Could you check a few things on this model? Use its own coordinates, in mm. A direction names the side the tool comes from. Coordinates: 2 decimals unless noted, no trailing zeros. Write each loop counter-clockwise with the first axis right and the second up, starting at its lowest first coordinate (ties: lowest second). Pieces come first, ordered by that corner, then holes.
```python
from build123d import *

# Parameters (mm, degrees)
F1_DEPTH = 1.2
F2_DEPTH = 2.2


with BuildPart() as f1:
    # F0 (on Top) → F1 (new body)
    with BuildSketch(Plane.XY):
        with BuildLine():
            ThreePointArc((-2.61423, 14.119491), (-10.150846, 10.145596), (-14.120842, 2.606925))
            Line((-14.120842, 2.606925), (-12.54888, 2.308583))
            ThreePointArc((-12.54888, 2.308583), (-12.746063, 0.003032), (-12.549977, -2.302612))
            Line((-12.549977, -2.302612), (-14.122546, -2.597676))
            ThreePointArc((-14.122546, -2.597676), (-10.138682, -10.128644), (-2.611663, -14.119966))
            Line((-2.611663, -14.119966), (-2.320738, -12.546638))
            ThreePointArc((-2.320738, -12.546638), (0.002028, -12.751949), (2.324728, -12.545899))
            Line((2.324728, -12.545899), (2.616123, -14.119141))
            ThreePointArc((2.616123, -14.119141), (10.123734, -10.218797), (14.094074, -2.747967))
            Line((14.094074, -2.747967), (12.522112, -2.449625))
            ThreePointArc((12.522112, -2.449625), (12.759115, -0.023547), (12.531068, 2.40339))
            Line((12.531068, 2.40339), (14.103637, 2.698454))
            ThreePointArc((14.103637, 2.698454), (10.129638, 10.19315), (2.610249, 14.120228))
            Line((2.610249, 14.120228), (2.319324, 12.546899))
            ThreePointArc((2.319324, 12.546899), (-0.001785, 12.754501), (-2.322835, 12.54625))
            Line((-2.322835, 12.54625), (-2.61423, 14.119491))
        make_face()
    extrude(amount=F1_DEPTH)

    # F0 (on Top) → F2 (join)
    with BuildSketch(Plane.XY):
        with BuildLine():
            Line((-12.54888, 2.308583), (-14.120842, 2.606925))
            ThreePointArc((-14.120842, 2.606925), (-14.353052, 0.0047), (-14.122546, -2.597676))
            Line((-14.122546, -2.597676), (-12.549977, -2.302612))
            ThreePointArc((-12.549977, -2.302612), (-12.746063, 0.003032), (-12.54888, 2.308583))
        make_face()
        with BuildLine():
            ThreePointArc((2.610249, 14.120228), (-0.002024, 14.357977), (-2.61423, 14.119491))
            Line((-2.61423, 14.119491), (-2.322835, 12.54625))
            ThreePointArc((-2.322835, 12.54625), (-0.001785, 12.754501), (2.319324, 12.546899))
            Line((2.319324, 12.546899), (2.610249, 14.120228))
        make_face()
        with BuildLine():
            ThreePointArc((14.094074, -2.747967), (14.356041, -0.025208), (14.103637, 2.698454))
            Line((14.103637, 2.698454), (12.531068, 2.40339))
            ThreePointArc((12.531068, 2.40339), (12.759115, -0.023547), (12.522112, -2.449625))
            Line((12.522112, -2.449625), (14.094074, -2.747967))
        make_face()
        with BuildLine():
            Line((-2.320738, -12.546638), (-2.611663, -14.119966))
            ThreePointArc((-2.611663, -14.119966), (0.002266, -14.349251), (2.616123, -14.119141))
            Line((2.616123, -14.119141), (2.324728, -12.545899))
            ThreePointArc((2.324728, -12.545899), (0.002028, -12.751949), (-2.320738, -12.546638))
        make_face()
    extrude(amount=F2_DEPTH)


solid = f1.part
```
1. On a 3-axis mill with a long thin cutter (end or side, diameter ignored), from which of +Z, -Z, +X, -X, +Y, -Y can I reach the whole of each face in a straight line? I mean faces 4 (the face through (13.297, -2.597, 1.693)), 5 (the face through (2.463, 13.323, 1.693)), 6 (the face through (-13.324, 2.456, 1.693)), 7 (the face through (-0.03, -14.35, 1.08)), 8 (the face through (12.76, 0.01, 1.69)). Say none if no direction works.
Verdict:
face 4: +Z, -Y
face 5: +Z, +X
face 6: +Z, +Y
face 7: +Z, -Z, -Y
face 8: +Z
2. I want a section at A-A on z = 1.75. Please give me the cut outline in (x, y), plus the area to 3 significant figures.
Verdict:
outline: (-14.12, -2.6) - (-12.55, -2.3) arc R13.62 cw to (-12.55, 2.31) - (-14.12, 2.61) arc R14.75 ccw to start; (-2.61, -14.12) arc R14.99 ccw to (2.62, -14.12) - (2.32, -12.55) arc R13.22 cw to (-2.32, -12.55) - close; (-2.61, 14.12) - (-2.32, 12.55) arc R13.06 cw to (2.32, 12.55) - (2.61, 14.12) arc R14.45 ccw to start; (12.52, -2.45) - (14.09, -2.75) arc R14.55 ccw to (14.1, 2.7) - (12.53, 2.4) arc R12.78 cw to start
area: 32.1 mm2
3. If we mould it in two halves opening along Y, with no side actions, what happens to faces 1 (the face through (-2.464, -13.322, 1.693)), 2 (the face through (-13.347, -2.452, 1.693)), 3 (the face through (0, -13, 2.2))? For each: pulls with the +Y half, pulls with the -Y half, needs draft (parallel to the pull), parting line crosses it, or undercut.
Verdict:
face 1: undercut
face 2: pulls with the -Y half
face 3: needs draft
4. Please list where these lines run through material, in increasing order: line 1 along Z through (x, y) = (-6.75, -8.25); line 2 along X through (y, z) = (-1.5, 1.5); line 3 along X through (y, z) = (0.25, 0.2).
Verdict:
line 1: z = 0 to 1.2
line 2: x = -14.28 to -12.66, 12.67 to 14.28
line 3: x = -14.35 to 14.35
5. I want a section at D-D on x = -10.25. Please give me the cut outline in (y, z).
Verdict:
outline: (-10.02, 0) - (10.05, 0) - (10.05, 1.2) - (-10.02, 1.2) - close
6. I want a section at C-C on y = -4. Please give me the cut outline in (x, z).
Verdict:
outline: (-13.78, 0) - (13.8, 0) - (13.8, 1.2) - (-13.78, 1.2) - close
7. For pin 1 (12 mm diameter, centred on x = 10.5, y = 1.5, fed in from +Z); pin 2 (1.5 mm diameter, centred on x = 6, y = 7, fed in from +Z), each with a flat end and sliding along its axis, tell me the tip position at first contact or that it passes through.
Verdict:
pin 1: stops at z = 2.2
pin 2: stops at z = 1.2
8. I want a section at B-B on x = 1.5. Please give me the cut outline in (y, z), plus the area to 3 significant figures.
Verdict:
outline: (-14.27, 0) - (14.28, 0) - (14.28, 2.2) - (12.67, 2.2) - (12.67, 1.2) - (-12.67, 1.2) - (-12.67, 2.2) - (-14.27, 2.2) - close
area: 37.5 mm2
